from build123d import *

# Parameters (mm, degrees)
F1_DEPTH = 2.286
F2_DEPTH = 2.286


with BuildPart() as f1:
    # F0 (on Front) → F1 (new body)
    with BuildSketch(Plane.XZ):
        Polygon((39.280557, 15.288984), (38.11859, 17.693268), (-63.09732, -31.223414), (-67.924149, -35.039101), (-61.935353, -33.627699), align=None)
    extrude(amount=F1_DEPTH)

    # F1_face (on face) → F2 (join)
    with BuildSketch(Plane(origin=(-13.27206, -2.286, -8.626268), x_dir=(1, 0, 0), z_dir=(0, -1, 0))):
        Polygon((-48.663293, -25.001431), (52.552618, 23.915252), (51.39065, 26.319536), (-49.82526, -22.597146), (-54.652089, -26.412833), align=None)
    extrude(amount=-F2_DEPTH)


solid = f1.part
Check sheet for the modelled part. Datum: model origin and axes. Units: mm. Give positions to 0.01 mm unless a question says otherwise; leave off trailing zeros. Write each loop counter-clockwise with the first axis right and the second up, starting at its lowest first coordinate (ties: lowest second). Pieces come first, ordered by that corner, then holes. Notation, with made-up numbers: (45, 76.5) -> (49, 76.5) arc R18 ccw to (49, 94.5) -> close; hole circle Ø7 at (40.25, 57.5). An arc over 180 degrees is marked (long way). One line per item, written item: value. Start each with the question number.
Item 1: Section check C-C on z = -3. Record the cut outline in (x, y), then the cut area to 3 significant figures.
Item 2: Section check B-B on x = -12. Record the cut outline in (y, z), then the cut area to 3 significant figures.
Item 3: Material ranges on probe 1 along Z at (x, y) = (-24.5, -1.15); probe 2 along X at (y, z) = (-0.35, 1); probe 3 along X at (y, z) = (-0.25, -24), recorded low to high. Write a range as from..to.
Item 4: Section check A-A on y = -0.8. Record the cut outline in (x, z), then the cut area to 3 significant figures.
Results list:
1. outline: (-4.7, -2.29) -> (1.44, -2.29) -> (1.44, 0) -> (-4.7, 0) -> close
1. area: 14.0 mm²
2. outline: (-2.29, -9.49) -> (0, -9.49) -> (0, -6.53) -> (-2.29, -6.53) -> close
2. area: 6.78 mm²
3. probe 1: -15.54..-12.57
3. probe 2: 3.58..9.71
3. probe 3: -48.15..-42.01
4. outline: (-67.92, -35.04) -> (-61.94, -33.63) -> (39.28, 15.29) -> (38.12, 17.69) -> (-63.1, -31.22) -> close
4. area: 308 mm²
